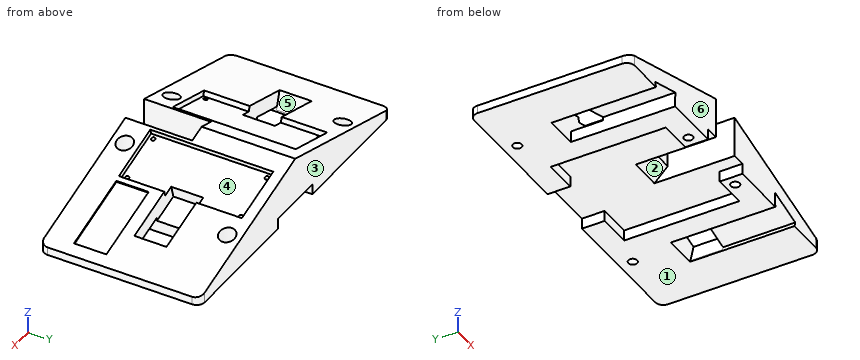
Solid Edge part; units mm, degrees
sketch "Sketch1" plane through (0, 0, 0) normal (0, 0, 1) x (1, 0, 0)
  line L0 (-61, 30) -> (61, 30)
  line L1 (61, 30) -> (61, -30)
  line L2 (61, -30) -> (-61, -30)
  line L3 (-61, -30) -> (-61, 30)
  dimension "D1" = 61
  dimension "D2" = 61
extrude "Protrusion1" add sketch "Sketch1" along normal blind 26
fillet "Redondeo_1" radius 3 4 edges at (61, 30, 13) (61, -30, 13) (-61, -30, 13) (-61, 30, 13)
sketch "Sketch2" plane through (0, 0, 26) normal (0, 0, 1) x (-1, 0, 0)
  circle A0 centre (15, 25) radius 1.65
  circle A1 centre (39, -25) radius 1.65
  circle A2 centre (-35, -25) radius 1.65
  circle A3 centre (-15, 25) radius 1.65
extrude "Cutout1" cut sketch "Sketch2" against normal up to next
sketch "Sketch3" plane through (0, 0, 26) normal (0, 0, 1) x (-1, 0, 0)
  circle A0 centre (-15, 25) radius 3
  circle A1 centre (15, 25) radius 3
  circle A2 centre (-35, -25) radius 3
  circle A3 centre (39, -25) radius 3
extrude "VaciadoExtruido_30" cut sketch "Sketch3" against normal blind 22
sketch "Sketch4" plane through (0, -30, 13) normal (0, -1, 0) x (-1, 0, 0)
  line L0 (0, -8) -> (-61, 10)
  line L1 (0, -8) -> (61, 10)
  dimension "D1" = 61
extrude "Cutout2" cut sketch "Sketch4" against normal up to next material side at (30.5142, -30, 12.048)
sketch "Sketch5" plane through (31.3143, 0, 11.7597) normal (0.283, 0, 0.9591) x (-0.9591, 0, 0.283)
  line L0 (4.1492, 20) -> (4.1492, -26)
  line L1 (4.1492, -26) -> (25.1492, -26)
  line L2 (25.1492, -26) -> (25.1492, 20)
  line L3 (25.1492, 20) -> (4.1492, 20)
  dimension "D1" = 4.1492
  dimension "D2" = 25.1492
extrude "Cutout3" cut sketch "Sketch5" against normal blind 2
sketch "Sketch6" plane through (31.3143, 0, 11.7597) normal (0.283, 0, 0.9591) x (-0.9591, 0, 0.283)
  line L0 (-15.8508, 3) -> (-15.8508, -9)
  line L1 (-15.8508, -9) -> (8.1492, -9)
  line L2 (8.1492, 3) -> (8.1492, -9)
  line L3 (-15.8508, 3) -> (8.1492, 3)
  dimension "D1" = 15.8508
  dimension "D2" = 15.8508
extrude "VaciadoExtruido_32" cut sketch "Sketch6" against normal blind 7
sketch "Sketch7" plane through (16.0737, 3, 14.1717) normal (0.283, 0, 0.9591) x (-0.9591, 0, 0.283)
  circle A0 centre (-9.4009, 21.25) radius 0.75
  circle A1 centre (8.0991, 21.25) radius 0.75
  circle A2 centre (8.0991, -21.25) radius 0.75
  circle A3 centre (-9.4009, -21.25) radius 0.75
extrude "VaciadoExtruido_33" cut sketch "Sketch7" against normal blind 4
sketch "Sketch8" plane through (32, -30, 9.6148) normal (0, -1, 0) x (-1, 0, 0)
  line L0 (-12.3707, 9.6148) -> (-0.0681, 9.6148)
  line L1 (-0.0681, 9.6148) -> (0, 4.0632)
  line L2 (-12.8868, 7.8658) -> (0, 4.0632)
  line L3 (-12.3707, 9.6148) -> (-12.8868, 7.8658)
extrude "Cutout4" cut sketch "Sketch8" against normal up to surface (39 mm away)
mirror "Mirror1" about plane through (0, 0, 0) normal (1, 0, 0) of "Cutout3", "VaciadoExtruido_32", "VaciadoExtruido_33", "Cutout4"
sketch "Sketch9" plane through (31.3143, 0, 11.7597) normal (0.283, 0, 0.9591) x (-0.9591, 0, 0.283)
  line L0 (-26.1597, 19.8186) -> (2.081, 19.8186)
  line L1 (2.081, 19.8186) -> (2.081, 7.703)
  line L2 (2.081, 7.703) -> (-26.1597, 7.703)
  line L3 (-26.1597, 7.703) -> (-26.1597, 19.8186)
extrude "VaciadoExtruido_38" cut sketch "Sketch9" against normal blind 0.5
sketch "Sketch10" plane through (0, 0, 0) normal (0, 0, -1) x (1, 0, 0)
  line L0 (-23.5, -21.5) -> (-23.5, 21.5)
  line L1 (23.5, 21.5) -> (-23.5, 21.5)
  line L2 (23.5, -21.5) -> (23.5, 21.5)
  line L3 (-23.5, -21.5) -> (23.5, -21.5)
  dimension "D1" = 23.5
  dimension "D2" = 23.5
extrude "VaciadoExtruido_39" cut sketch "Sketch10" against normal blind 4
sketch "Sketch11" plane through (0, 0, 0) normal (0, 0, -1) x (1, 0, 0)
  line L0 (-11, 30) -> (-11, -30)
  line L1 (-11, -30) -> (11, -30)
  line L2 (11, -30) -> (11, 30)
  line L3 (11, 30) -> (-11, 30)
extrude "Cutout9" cut sketch "Sketch11" against normal up to surface (4 mm away)
sketch "Sketch12" plane through (0, -30, 9) normal (0, -1, 0) x (1, 0, 0)
  line L0 (-6, 14) -> (6, 14)
  line L1 (6, 14) -> (6, -9)
  line L2 (6, -9) -> (-6, -9)
  line L3 (-6, -9) -> (-6, 14)
  dimension "D1" = 6
  dimension "D2" = 6
extrude "VaciadoExtruido_41" cut sketch "Sketch12" against normal blind 25
chamfer "Chaflán_2" distance 5 angle 45 1 edges at (0, -5, 4)
properties material "Aluminum, 2024-T4"
For this review, take the finished solid that the model builds, in its own axes (mm). Face numbers are marked on the shaded views. A direction names the side the tool comes from. Round coordinates to 2 decimals unless told otherwise and drop trailing zeros. Order: outer loops, then holes, each group sorted by start corner. A loop starts at its lowest first (then second) coordinate and runs counter-clockwise, first axis right, second up. Notation, with made-up numbers: M 39.5,78 L 43.5,78 A23 cw 43.5,114 Z; hole C 22.5,-11.5 d2. An arc over 180 degrees is marked long. Use a Markdown table: item, result. Add a question column.
Item 1: Mouldability with a two-part tool opening along Y and no side actions: class the marked faces 1, 2, 3 and 4 as released by +Y, released by -Y, zero draft, split by the parting line, or undercut.
Item 2: To check wall thickness, follow line 1 along Y through (x, z) = (35, 6); line 2 along Y through (x, z) = (35, 2); line 3 along Y through (x, z) = (21, 3.25). State the ranges of each line that lie inside material, in increasing order.
Item 3: Insertion check: pin 1 (12 mm diameter, centred on x = -37, y = -2.5, fed in from +Z); pin 2 (5 mm diameter, centred on x = -15, y = -25, fed in from +Z); pin 3 (2 mm diameter, centred on x = -0.5, z = 5, fed in from -Y); pin 4 (2.5 mm diameter, centred on x = 35, y = 25, fed in from -Z). Each pin has a flat end and moves straight along its axis. Give the tip position at first contact, or say it passes through.
Item 4: Add section B-B, the plane x = -39. Give the boundary of the cut face in (y, z), then the cut area to 3 significant figures.
Item 5: Add section D-D, the plane x = -15. Give the boundary of the cut face in (y, z).
Item 6: Add section C-C, the plane y = 19. Give the boundary of the cut face in (x, z), then the cut area to 3 significant figures.
Item 7: Tool access review of the marked faces 5 and 6: name each direction out of +Z, -Z, +X, -X, +Y, -Y from which nothing blocks a thin tool from reaching the whole face with its end or side.
Geometry results:
| question | item | result |
|---|---|---|
| 1 | face 1 | zero draft |
| 1 | face 2 | released by -Y |
| 1 | face 3 | released by +Y |
| 1 | face 4 | undercut |
| 2 | line 1 | y = -30 to -3, 9 to 22, 28 to 30 |
| 2 | line 2 | y = 9 to 23.35, 26.65 to 30 |
| 2 | line 3 | y = -30 to -21.5, 21.5 to 30 |
| 3 | pin 1 | stops at z = 11.85 |
| 3 | pin 2 | stops at z = 4 |
| 3 | pin 3 | stops at y = -2 |
| 3 | pin 4 | passes through |
| 4 | outline | M -30,3.49 L -3,3.49 L -3,9.49 L -30,9.49 Z; M 9,0 L 23.35,0 L 23.35,4 L 22,4 L 22,9.49 L 9,9.49 Z; M 26.65,0 L 30,0 L 30,9.49 L 28,9.49 L 28,4 L 26.65,4 Z |
| 4 | area | 315 mm² |
| 5 | outline | M -30,0 L -26.65,0 L -26.65,4 L -28,4 L -28,16.57 L -30,16.57 Z; M -23.35,0 L -21.5,0 L -21.5,4 L 21.5,4 L 21.5,0 L 30,0 L 30,16.57 L 26,16.57 L 26,14.49 L -20,14.49 L -20,16.57 L -22,16.57 L -22,4 L -23.35,4 Z |
| 6 | outline | M -61,0 L -23.5,0 L -23.5,4 L 23.5,4 L 23.5,0 L 61,0 L 61,3 L 27.33,12.93 L 26.77,11.02 L 6.63,16.96 L 7.19,18.88 L 0,21 L -7.19,18.88 L -6.63,16.96 L -26.77,11.02 L -27.33,12.93 L -61,3 Z |
| 6 | area | 1,190 mm² |
| 7 | face 5 | +Z |
| 7 | face 6 | +Z, -Z, +X, -X, -Y |
